Input: part model. Units: mm. Frame: model coordinates. A direction names the side the tool comes from. Give positions to 0.01 mm unless a question says otherwise; leave off trailing zeros. Loops run counter-clockwise (first coordinate to the right, second up) from the corner with the lowest first, then second, coordinate; pieces in that order, holes last. Notation, with made-up numbers: M 81.25,15.25 L 127.25,15.25 A25 ccw 127.25,34.25 Z; hole C 22.5,29.25 d2. An arc over 180 degrees is marked long. Return JSON: item names as keys, results as strings. Group by question number.
```python
from build123d import *

# Parameters (mm, degrees)
F0_R     = 457.2
F0_R_2   = 419.1
F0_R_3   = 361.95
F0_R_4   = 323.85
F1_DEPTH = 76.2
F2_R     = 419.1
F2_R_2   = 361.95
F3_DEPTH = 38.1
F4_DEPTH = 38.1
F5_R     = 323.85
F5_R_2   = 285.75
F6_DEPTH = 38.1
F7_R     = 323.85
F7_R_2   = 285.75
F8_DEPTH = 38.1


with BuildPart() as f1:
    # F0 (on Right) → F1 (new body)
    with BuildSketch(Plane.YZ):
        Circle(F0_R)
        Circle(F0_R_2, mode=Mode.SUBTRACT)
        Circle(F0_R_2)
        Circle(F0_R_3, mode=Mode.SUBTRACT)
        Circle(F0_R_3)
        Circle(F0_R_4, mode=Mode.SUBTRACT)
    extrude(amount=F1_DEPTH)

    # F2 (on face) → F3 (cut)
    with BuildSketch(Plane.YZ.offset(76.2)):
        Circle(F2_R)
        Circle(F2_R_2, mode=Mode.SUBTRACT)
    extrude(amount=-F3_DEPTH, mode=Mode.SUBTRACT)

    # F4 (add): a face of the model
    f4_faces = [f1.faces().sort_by_distance(p)[0] for p in [
        (76.2, -351.712508022, 0),
    ]]
    extrude(f4_faces, amount=F4_DEPTH)

    # F5 (on Right) → F6 (join)
    with BuildSketch(Plane.YZ):
        Circle(F5_R)
        Circle(F5_R_2, mode=Mode.SUBTRACT)
    extrude(amount=F6_DEPTH)

    # F7 (on face) → F8 (join)
    with BuildSketch(Plane.YZ.offset(114.3)):
        Circle(F7_R)
        Circle(F7_R_2, mode=Mode.SUBTRACT)
    extrude(amount=-F8_DEPTH)


solid = f1.part
```
Item 1: First-contact query: pin 1 Ø3 at (x, z) = (70.5, 97) entering from -Y; pin 2 Ø2 at (x, y) = (70.5, 122.5) entering from -Z; pin 3 Ø6 at (x, y) = (75, -304) entering from +Z. Flat tips, straight axial feed; report the tip coordinate or a pass-through.
Item 2: Section A-A, the plane y = 0. Return loops of the section in (x, z).
Item 3: Section C-C, the plane x = 55.5. Return loops of the section in (y, z).
Item 4: Reachability of faces 5 (the face through (38.1, -312, -184)), 6 (the face through (114.3, 266, 109)), 7 (the face through (38.1, -2, -286)) from +Z, -Z, +X, -X, +Y, -Y: full face, straight path, thin tool, end or side. Return the list, or none.
Item 5: Material intervals for line 1 (Z direction, x = 63, y = 0); line 2 (X direction, y = -206, z = 248); line 3 (Z direction, x = 106.5, y = 0), sorted ascending. Write a range as from..to.
Item 6: Pull-direction query (Y, two-part tool) for faces 1 (the face through (56.883, -42.159, 321.094)), 2 (the face through (0, -210, -197)), 3 (the face through (57.417, -90.853, -409.134)), 4 (the face through (37.567, -456.758, 20.102)); classes: pulls with the +Y half, pulls with the -Y half, needs draft (parallel to the pull), parting line crosses it, or undercut.
Answer below:
{
 "1": {"pin 1": "y = -447.11", "pin 2": "z = -440.76", "pin 3": "z = 344.14"},
 "2": {"outline": "M 0,-457.2 L 76.2,-457.2 L 76.2,-419.1 L 38.1,-419.1 L 38.1,-361.95 L 114.3,-361.95 L 114.3,-285.75 L 76.2,-285.75 L 76.2,-323.85 L 38.1,-323.85 L 38.1,-285.75 L 0,-285.75 Z; M 0,285.75 L 38.1,285.75 L 38.1,323.85 L 76.2,323.85 L 76.2,285.75 L 114.3,285.75 L 114.3,361.95 L 38.1,361.95 L 38.1,419.1 L 76.2,419.1 L 76.2,457.2 L 0,457.2 Z"},
 "3": {"outline": "C 0,0 d914.4; C 0,0 d723.9; hole C 0,0 d838.2; hole C 0,0 d647.7"},
 "4": {"face 5": "+X", "face 6": "+Z, -Z, +X, +Y, -Y", "face 7": "none"},
 "5": {"line 1": "-457.2..-419.1, -361.95..-323.85, 323.85..361.95, 419.1..457.2", "line 2": "0..38.1, 76.2..114.3", "line 3": "-361.95..-285.75, 285.75..361.95"},
 "6": {"face 1": "undercut", "face 2": "needs draft", "face 3": "undercut", "face 4": "parting line crosses it"}
}
